The listing builds one solid part. Answer for the finished solid, in the listing's coordinates (mm). A direction names the side the tool comes from. Give positions to 0.01 mm unless a question says otherwise; leave off trailing zeros. Order: outer loops, then holes, each group sorted by start corner. A loop starts at its lowest first (then second) coordinate and runs counter-clockwise, first axis right, second up. Notation, with made-up numbers: (64.5, -9.75) - (112.5, -9.75) arc R18 cw to (112.5, 3.25) - close; hole circle Ø5 at (71, 31.25). An arc over 180 degrees is marked (long way). Answer in a Markdown table with one row per item. Add a question column.
```python
from build123d import *

# Parameters (mm, degrees)
SKETCH1_W           = 120
SKETCH1_H           = 58
BOSS_EXTRUDE5_DEPTH = 5
SKETCH5_R           = 2.5
CUT_EXTRUDE2_DEPTH  = 5
SKETCH6_W           = 40
SKETCH6_H           = 6
BOSS_EXTRUDE6_DEPTH = 3
SKETCH7_R           = 11.25
CUT_EXTRUDE3_DEPTH  = 2
SKETCH8_R           = 4
CUT_EXTRUDE4_DEPTH  = 12
SKETCH9_R           = 5.1
CUT_EXTRUDE5_DEPTH  = 1.5
SKETCH10_R          = 1.75
CUT_EXTRUDE6_DEPTH  = 21.5
CHAMFER1_SIZE       = 40


with BuildPart() as part:
    # Sketch1 → Boss-Extrude5 (new body)
    with BuildSketch(Plane(origin=(0, 0, 0), x_dir=(1, 0, 0), z_dir=(0, 1, 0))):
        with Locations((60, 29)):
            Rectangle(SKETCH1_W, SKETCH1_H)
    extrude(amount=BOSS_EXTRUDE5_DEPTH)

    # Sketch5 → Cut-Extrude2 (cut)
    with BuildSketch(Plane(origin=(0, 5, 0), x_dir=(1, 0, 0), z_dir=(0, 1, 0))):
        with Locations(Location((10, 48, 0), (0, 0, 270))):
            Circle(SKETCH5_R)
        with Locations(Location((60, 48, 0), (0, 0, 270))):
            Circle(SKETCH5_R)
        with Locations(Location((110, 48, 0), (0, 0, 270))):
            Circle(SKETCH5_R)
    extrude(amount=-CUT_EXTRUDE2_DEPTH, mode=Mode.SUBTRACT)

    # Sketch6 → Boss-Extrude6 (add)
    with BuildSketch(Plane(origin=(0, 5, 0), x_dir=(1, 0, 0), z_dir=(0, 1, 0))):
        with Locations((35, 48)):
            Rectangle(SKETCH6_W, SKETCH6_H)
        with Locations((85, 48)):
            Rectangle(SKETCH6_W, SKETCH6_H)
    extrude(amount=BOSS_EXTRUDE6_DEPTH)

    # Sketch7 → Cut-Extrude3 (cut)
    with BuildSketch(Plane(origin=(0, 5, 0), x_dir=(1, 0, 0), z_dir=(0, 1, 0))):
        with Locations(Location((60, 13.85, 0), (0, 0, 270))):
            Circle(SKETCH7_R)
    extrude(amount=-CUT_EXTRUDE3_DEPTH, mode=Mode.SUBTRACT)

    # Sketch8 → Cut-Extrude4 (cut)
    with BuildSketch(Plane(origin=(0, 3, 0), x_dir=(1, 0, 0), z_dir=(0, 1, 0))):
        with Locations(Location((60, 13.85, 0), (0, 0, 270))):
            Circle(SKETCH8_R)
    extrude(amount=-CUT_EXTRUDE4_DEPTH, mode=Mode.SUBTRACT)

    # Sketch9 → Cut-Extrude5 (cut)
    with BuildSketch(Plane(origin=(0, 3, 0), x_dir=(1, 0, 0), z_dir=(0, 1, 0))):
        with Locations(Location((60, 13.85, 0), (0, 0, 270))):
            Circle(SKETCH9_R)
    extrude(amount=-CUT_EXTRUDE5_DEPTH, mode=Mode.SUBTRACT)

    # Sketch10 → Cut-Extrude6 (cut)
    with BuildSketch(Plane(origin=(0, 3, 0), x_dir=(1, 0, 0), z_dir=(0, 1, 0))):
        with Locations(Location((52, 13.85, 0), (0, 0, 270))):
            Circle(SKETCH10_R)
        with Locations(Location((60, 21.85, 0), (0, 0, 270))):
            Circle(SKETCH10_R)
        with Locations(Location((68, 13.85, 0), (0, 0, 270))):
            Circle(SKETCH10_R)
        with Locations(Location((60, 5.85, 0), (0, 0, 270))):
            Circle(SKETCH10_R)
    extrude(amount=-CUT_EXTRUDE6_DEPTH, mode=Mode.SUBTRACT)

    # Chamfer1
    chamfer1_edges = [part.edges().sort_by_distance(p)[0] for p in [
        (120, 2.5, 0),
        (0, 2.5, 0),
    ]]
    chamfer(chamfer1_edges, length=CHAMFER1_SIZE)


solid = part.part
```
(1) The mould has two halves that part along Z. Classify faces 4 (the face through (59.04, 2.54, -45.69)), 5 (the face through (85, 6, -45)), 6 (the face through (0, 2, -49)): +Z half, -Z half, draft (parallel to the pull), parting line (faces both ways), or undercut.
(2) Straight lines are drawn through the part: line 1 (X direction, y = 2.05, z = -48); line 2 (X direction, y = 1.1, z = -13.85); line 3 (Y direction, x = 50, z = -10). For each, find the intervals that lie inside material, in ascending order.
(3) For faces 1 (the face through (71.154, 4.014, -15.315)), 2 (the face through (35, 6, -51)), 3 (the face through (55, 6, -48)), determine the directions among +Z, -Z, +X, -X, +Y, -Y from which every point of the face is accessible in a straight line to the end or side of a thin tool.
(4) Find section D-D, the plane z = -13.85. Write down the section's boundary in (x, y).
(5) Find section A-A, the plane z = -48. Write down the section's boundary in (x, y).
(6) Find section B-B, the plane x = 110. Write down the section's boundary in (y, z).
(7) Each of these flat-tipped pins is pushed along its axis until it touches: P1, Ø2, axis at y = 5.5, z = -22.5, coming from the +X side; P2, Ø4, axis at x = 76.5, z = -6, coming from the +Y side; P3, Ø3.5, axis at x = 93, y = 6, coming from the +Z side; P4, Ø3, axis at x = 52, z = -13.85, coming from the +Y side (1 decimal). Where does it stop, or does it pass through?
(8) Find section C-C, the plane x = 31.5. Write down the section's boundary in (y, z), plus the area to 4 significant figures.
Answer key:
| question | item | result |
|---|---|---|
| 1 | face 4 | undercut |
| 1 | face 5 | +Z half |
| 1 | face 6 | draft |
| 2 | line 1 | 0 to 7.5, 12.5 to 57.5, 62.5 to 107.5, 112.5 to 120 |
| 2 | line 2 | 26.15 to 50.25, 53.75 to 56, 64 to 66.25, 69.75 to 93.85 |
| 2 | line 3 | 0 to 3 |
| 3 | face 1 | +Y |
| 3 | face 2 | -Z, +X, -X, +Y |
| 3 | face 3 | +Z, -Z, +Y |
| 4 | outline | (26.15, 0) - (50.25, 0) - (50.25, 3) - (48.75, 3) - (48.75, 5) - (26.15, 5) - close; (53.75, 0) - (56, 0) - (56, 1.5) - (54.9, 1.5) - (54.9, 3) - (53.75, 3) - close; (64, 0) - (66.25, 0) - (66.25, 3) - (65.1, 3) - (65.1, 1.5) - (64, 1.5) - close; (69.75, 0) - (93.85, 0) - (93.85, 5) - (71.25, 5) - (71.25, 3) - (69.75, 3) - close |
| 5 | outline | (0, 0) - (7.5, 0) - (7.5, 5) - (0, 5) - close; (12.5, 0) - (57.5, 0) - (57.5, 5) - (55, 5) - (55, 8) - (15, 8) - (15, 5) - (12.5, 5) - close; (62.5, 0) - (107.5, 0) - (107.5, 5) - (105, 5) - (105, 8) - (65, 8) - (65, 5) - (62.5, 5) - close; (112.5, 0) - (120, 0) - (120, 5) - (112.5, 5) - close |
| 6 | outline | (0, -58) - (5, -58) - (5, -50.5) - (0, -50.5) - close; (0, -45.5) - (5, -45.5) - (5, -30) - (0, -30) - close |
| 7 | P1 | x = 103.37 |
| 7 | P2 | y = 5 |
| 7 | P3 | z = -11.56 |
| 7 | P4 | through |
| 8 | outline | (0, -58) - (5, -58) - (5, -51) - (8, -51) - (8, -45) - (5, -45) - (5, -8.5) - (0, -8.5) - close |
| 8 | area | 265.5 mm² |
